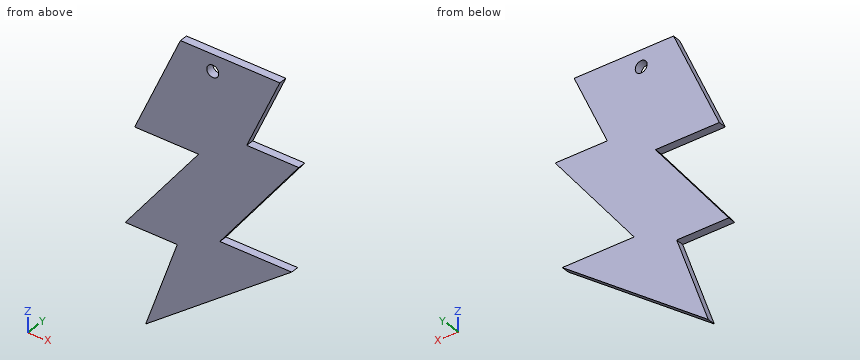
from build123d import *

# Parameters (mm, degrees)
F0_R     = 1.905
F1_DEPTH = 2.54
F2_DEPTH = 152


# Not quite as in the source:
# - an extrude ends at something that could not be found from the text; its depth is read off the source's solid


with BuildPart() as f1:
    # F0 (on Front) → F1 (new body)
    with BuildSketch(Plane.XZ):
        Polygon((-10.5372872204, 53.1882047653), (0, 76.7774991782), (-31.6092483094, 76.7774991782), (-46.1633428931, 44.156242162), (-25.8414391428, 44.156242162), (-49.1739995778, 13.5479401797), (-32.6154083014, 13.5479401797), (-42.6509156823, -15.0532610714), (3.763313638, 20.0710203499), (-19.0674699843, 20.0710203499), (6.0213026591, 53.1882047653), align=None)
        with Locations((-21.3299991501, 71.5437866839)):
            Circle(F0_R, mode=Mode.SUBTRACT)
    extrude(amount=F1_DEPTH)

    # F0 (on Front) → F2 (cut, through all)
    with BuildSketch(Plane.XZ):
        with Locations((-21.3299991501, 71.5437866839)):
            Circle(F0_R)
    extrude(amount=-F2_DEPTH, mode=Mode.SUBTRACT)


solid = f1.part
Geometry: final body of the model. Coordinates: model frame, mm. Round coordinates to 2 decimals unless told otherwise and drop trailing zeros. Order: outer loops, then holes, each group sorted by start corner. A loop starts at its lowest first (then second) coordinate and runs counter-clockwise, first axis right, second up.
Q1. Material intervals for probe 1 along Z at (x, y) = (-10, -1.9); probe 2 along Z at (x, y) = (1.5, -2); probe 3 along Z at (x, y) = (-21.33, -0.7), sorted ascending.
Result sheet:
probe 1: z = 9.66 to 20.07, 32.04 to 53.19, 54.39 to 76.78
probe 2: z = 18.36 to 20.07, 47.22 to 53.19
probe 3: z = 1.08 to 69.64, 73.45 to 76.78
Q2. Section C-C, the plane x = -5. Output: boundary loops of the cut face in (y, z).
Result sheet:
outline: (-2.54, 13.44) - (0, 13.44) - (0, 20.07) - (-2.54, 20.07) - close; (-2.54, 38.64) - (0, 38.64) - (0, 53.19) - (-2.54, 53.19) - close; (-2.54, 65.58) - (0, 65.58) - (0, 76.78) - (-2.54, 76.78) - close
Q3. Pin query (flat end, axial travel): pin 1 (5 mm diameter, centred on x = -6, z = 9.5, fed in from -Y); pin 2 (1 mm diameter, centred on x = -39, y = -1.5, fed in from +Z); pin 3 (1 mm diameter, centred on y = -0.5, z = 51.5, fed in from -X); pin 4 (1.3 mm diameter, centred on x = -43.5, y = -1, fed in from -Z). Return the tip coordinate at first contact, or that it passes through.
Result sheet:
pin 1: passes through
pin 2: stops at z = 61.33
pin 3: stops at x = -43.11
pin 4: stops at z = 13.55
Q4. Section D-D, the plane x = -12. Output: boundary loops of the cut face in (y, z), and give its area (3 significant figures).
Result sheet:
outline: (-2.54, 8.14) - (0, 8.14) - (0, 20.07) - (-2.54, 20.07) - close; (-2.54, 29.4) - (0, 29.4) - (0, 76.78) - (-2.54, 76.78) - close
area: 151 mm2
Q5. Section B-B, the plane y = -1.55. Output: boundary loops of the cut face in (x, z) (1 decimal), and give its area (3 significant figures).
Result sheet:
outline: (-49.2, 13.5) - (-32.6, 13.5) - (-42.7, -15.1) - (3.8, 20.1) - (-19.1, 20.1) - (6, 53.2) - (-10.5, 53.2) - (0, 76.8) - (-31.6, 76.8) - (-46.2, 44.2) - (-25.8, 44.2) - close; hole circle Ø3.8 at (-21.3, 71.5)
area: 2,460 mm2
Q6. Section A-A, the plane x = -21.33. Output: boundary loops of the cut face in (y, z).
Result sheet:
outline: (-2.54, 1.08) - (0, 1.08) - (0, 69.64) - (-2.54, 69.64) - close; (-2.54, 73.45) - (0, 73.45) - (0, 76.78) - (-2.54, 76.78) - close
